The model under review builds one solid part; all positions refer to its coordinate system, in mm. Round coordinates to 2 decimals unless told otherwise and drop trailing zeros. Order: outer loops, then holes, each group sorted by start corner. A loop starts at its lowest first (then second) coordinate and runs counter-clockwise, first axis right, second up. Notation, with made-up numbers: M 23.5,72.25 L 56.5,72.25 A32 cw 56.5,108.25 Z; hole C 10.25,-23 d6. An arc over 180 degrees is marked long. One line per item, written item: value. Start each with the question number.
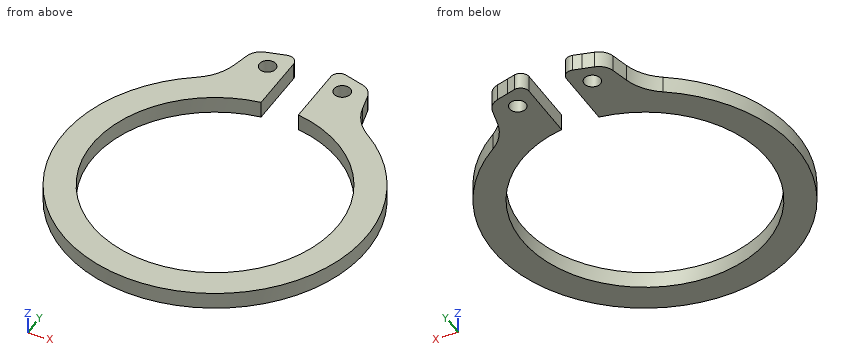
from build123d import *

# Parameters (mm, degrees)
SKETCH_1_R      = 0.491728838
EXTRUDE_1_DEPTH = 1


with BuildPart() as part:
    # 草图1 → 凸台-拉伸1 (new body)
    with BuildSketch(Plane.XY):
        with BuildLine():
            Line((1.748834408, 11.402867185), (2.236845371, 11.271018751))
            Line((2.236845371, 11.271018751), (2.906504263, 11.090093561))
            ThreePointArc((2.906504263, 11.090093561), (3.363858628, 10.820566678), (3.618817735, 10.354934194))
            Line((3.618817735, 10.354934194), (3.861047435, 9.33106424))
            ThreePointArc((3.861047435, 9.33106424), (4.311482707, 8.317586053), (5.09935285, 7.537015358))
            ThreePointArc((5.09935285, 7.537015358), (0, -9.1), (-5.09935285, 7.537015358))
            ThreePointArc((-5.09935285, 7.537015358), (-4.311482707, 8.317586053), (-3.861047435, 9.33106424))
            Line((-3.861047435, 9.33106424), (-3.618817735, 10.354934194))
            ThreePointArc((-3.618817735, 10.354934194), (-3.363858628, 10.820566678), (-2.906504263, 11.090093561))
            Line((-2.906504263, 11.090093561), (-2.236845371, 11.271018751))
            Line((-2.236845371, 11.271018751), (-1.748834408, 11.402867185))
            ThreePointArc((-1.748834408, 11.402867185), (-1.314453823, 11.317166281), (-1.118422685, 10.920173925))
            Line((-1.118422685, 10.920173925), (-1.118422685, 9.031009395))
            Line((-1.118422685, 9.031009395), (-1.118422685, 7.264408489))
            ThreePointArc((-1.118422685, 7.264408489), (0, -7.35), (1.118422685, 7.264408489))
            Line((1.118422685, 7.264408489), (1.118422685, 9.031009395))
            Line((1.118422685, 9.031009395), (1.118422685, 10.920173925))
            ThreePointArc((1.118422685, 10.920173925), (1.314453823, 11.317166281), (1.748834408, 11.402867185))
        make_face()
        with Locations((2.236845371, 10.095934401)):
            Circle(SKETCH_1_R, mode=Mode.SUBTRACT)
        with Locations(Location((-2.236845371, 10.095934401, 0), (0, 0, 180))):
            Circle(SKETCH_1_R, mode=Mode.SUBTRACT)
    extrude(amount=EXTRUDE_1_DEPTH)


solid = part.part
Item 1: Consider section C-C, the plane z = 0.45. Give the boundary of the cut face in (x, y).
Item 2: Consider section B-B, the plane x = -4.25. Give the boundary of the cut face in (y, z).
Item 3: Wall thickness on L1, parallel to X at y = 0, z = 0.55; L2, parallel to X at y = 4.75, z = 0.35; L3, parallel to Y at x = -3.5, z = 0.85: over which ranges is each line inside the solid? List them lowest first.
Item 4: Consider section D-D, the plane x = 0. Give the boundary of the cut face in (y, z), then the cut area to 3 significant figures.
Item 5: Consider section A-A, the plane y = -3.5. Give the boundary of the cut face in (x, z), then the cut area to 3 significant figures.
Computed:
1. outline: M -5.1,7.54 A9.1 ccw long 5.1,7.54 A3 cw 3.86,9.33 L 3.62,10.35 A1 ccw 2.91,11.09 L 1.75,11.4 A0.5 ccw 1.12,10.92 L 1.12,7.26 A7.35 cw long -1.12,7.26 L -1.12,10.92 A0.5 ccw -1.75,11.4 L -2.91,11.09 A1 ccw -3.62,10.35 L -3.86,9.33 A3 cw Z; hole C -2.24,10.1 d0.98; hole C 2.24,10.1 d0.98
2. outline: M -8.05,0 L -6,0 L -6,1 L -8.05,1 Z; M 6,0 L 8.41,0 L 8.41,1 L 6,1 Z
3. L1: x = -9.1 to -7.35, 7.35 to 9.1
3. L2: x = -7.76 to -5.61, 5.61 to 7.76
3. L3: y = -8.4 to -6.46, 6.46 to 10.64
4. outline: M -9.1,0 L -7.35,0 L -7.35,1 L -9.1,1 Z
4. area: 1.75 mm^2
5. outline: M -8.4,0 L -6.46,0 L -6.46,1 L -8.4,1 Z; M 6.46,0 L 8.4,0 L 8.4,1 L 6.46,1 Z
5. area: 3.87 mm^2
